Work out the finished part from the listing and answer in its coordinate system (mm). Face numbers are marked on the shaded views. Give positions to 0.01 mm unless a question says otherwise; leave off trailing zeros. Order: outer loops, then holes, each group sorted by start corner. A loop starts at its lowest first (then second) coordinate and runs counter-clockwise, first axis right, second up.
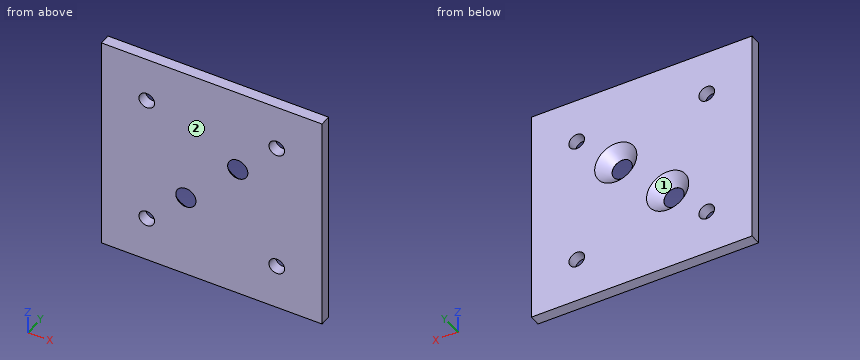
```python
from build123d import *

# Parameters (mm, degrees)
CROQUIS1_W                                  = 60
CROQUIS1_H                                  = 60
CROQUIS1_R                                  = 2.125
CROQUIS1_R_2                                = 0.5
SALIENTE_EXTRUIR1_DEPTH                     = 3
AVELLANADO_PARA_TORNILLO_CON_CABEZA_2_COUNT = 2
AVELLANADO_PARA_TORNILLO_CON_CABEZA_2_PITCH = 19.999930309


with BuildPart() as part:
    # Croquis1 → Saliente-Extruir1 (new body)
    with BuildSketch(Plane(origin=(0, 0, 0), x_dir=(1, 0, 0), z_dir=(0, 1, 0))):
        with Locations((30, 30)):
            Rectangle(CROQUIS1_W, CROQUIS1_H)
        with Locations((12.32233047, 47.67766953)):
            Circle(CROQUIS1_R, mode=Mode.SUBTRACT)
        with Locations((12.32233047, 12.32233047)):
            Circle(CROQUIS1_R, mode=Mode.SUBTRACT)
        with Locations((47.67766953, 12.32233047)):
            Circle(CROQUIS1_R, mode=Mode.SUBTRACT)
        with Locations((47.67766953, 47.67766953)):
            Circle(CROQUIS1_R, mode=Mode.SUBTRACT)
        with Locations((22.966364616, 37.108303123)):
            Circle(CROQUIS1_R_2, mode=Mode.SUBTRACT)
        with Locations((37.071067812, 22.928932188)):
            Circle(CROQUIS1_R_2, mode=Mode.SUBTRACT)
    extrude(amount=SALIENTE_EXTRUIR1_DEPTH)

    # Croquis8 → Avellanado para tornillo con cabeza avellanada de clavija hexagonal de M53 (revolve, cut)
    with BuildSketch(Plane(origin=(22.966364616, 3, -37.108303123), x_dir=(0, 0, 1), z_dir=(1, 0, 0))):
        Polygon((0, 0), (0, 3), (2.75, 3), (2.75, 2.985), (5.735, 0), align=None)
    avellanado_para_tornillo_con_cabeza_avel = revolve(axis=Axis((22.966364616, 9.35, -37.108303123), (0, -1, 0)), mode=Mode.SUBTRACT)

    # Avellanado para tornillo con cabeza  2: Avellanado para tornillo con cabeza avellanada de clavija hexagonal de M53 ×2
    with Locations(*[Vector(0.705237617, 0, 0.708971017) * (i * AVELLANADO_PARA_TORNILLO_CON_CABEZA_2_PITCH) for i in range(1, AVELLANADO_PARA_TORNILLO_CON_CABEZA_2_COUNT)]):
        add(avellanado_para_tornillo_con_cabeza_avel, mode=Mode.SUBTRACT)


solid = part.part
```
1. The mould has two halves that part along X. Classify the marked faces 1 and 2: pulls with the +X half, pulls with the -X half, needs draft (parallel to the pull), parting line crosses it, or undercut.
Findings below:
face 1: undercut
face 2: needs draft
2. The part is cut by section B-B (z = -48.5). Write down the section's boundary in (x, y).
Findings below:
outline: (0, 0) - (10.36, 0) - (10.36, 3) - (0, 3) - close; (14.28, 0) - (45.72, 0) - (45.72, 3) - (14.28, 3) - close; (49.64, 0) - (60, 0) - (60, 3) - (49.64, 3) - close
3. Straight lines are drawn through the part: probe 1 along Z at (x, y) = (13, 0.5); probe 2 along X at (y, z) = (1.35, -48); probe 3 along X at (y, z) = (1.7, -47). For each, find the intervals that lie inside material, in ascending order.
Findings below:
probe 1: z = -60 to -49.69, -45.66 to -14.34, -10.31 to 0
probe 2: x = 0 to 10.22, 14.42 to 45.58, 49.78 to 60
probe 3: x = 0 to 10.31, 14.34 to 45.66, 49.69 to 60
4. The part is cut by section A-A (y = 2.4). Write down the section's boundary in (x, z) (3 decimals).
Findings below:
outline: (0, -60) - (60, -60) - (60, 0) - (0, 0) - close; hole circle Ø4.25 at (12.322, -47.678); hole circle Ø4.25 at (12.322, -12.322); hole circle Ø10.27 at (22.966, -37.108); hole circle Ø10.27 at (37.071, -22.929); hole circle Ø4.25 at (47.678, -47.678); hole circle Ø4.25 at (47.678, -12.322)
